The listing builds one solid part. Answer for the finished solid, in the listing's coordinates (mm). A direction names the side the tool comes from. Give positions to 0.01 mm unless a question says otherwise; leave off trailing zeros. Order: outer loops, then holes, each group sorted by start corner. A loop starts at its lowest first (then second) coordinate and runs counter-clockwise, first axis right, second up. Notation, with made-up numbers: (56.5, 22.25) - (92.5, 22.25) arc R23 cw to (92.5, 36.25) - close; hole circle Ø4 at (75, 57.5). An arc over 180 degrees is marked (long way). Answer as a JSON object with one key per item and string values. Group by question number.
Q1. Given pin 1 (6 mm diameter, centred on x = 10, y = 13, fed in from +Z); pin 2 (10 mm diameter, centred on x = 5.5, z = 16, fed in from +Y); pin 3 (8 mm diameter, centred on x = 14.5, z = 6.5, fed in from +Y), each flat-ended and moving along its own axis, determine where each tip first touches the part or whether it passes through.
Q2. Consider line 1 (Z direction, x = 31.5, y = 15); line 2 (Z direction, x = 16, y = 14); line 3 (X direction, y = 23.5, z = 33.5). Determine where each line is inside the solid, lowest interval first.
Q3. For faces 1 (the face through (0, 25, 25)), 2 (the face through (15, 20, 0)), determine the directions among +Z, -Z, +X, -X, +Y, -Y from which every point of the face is accessible in a straight line to the end or side of a thin tool.
Q4. A cutting plane is placed at B-B, the plane y = 38.5. Give the vertices of the cut face in (x, z), and give its area (3 significant figures).
Q5. A cutting plane is placed at A-A, the plane x = 21.5. Give the vertices of the cut face in (y, z).
Q6. The mould has two halves that part along Y. Classify faces 3 (the face through (22.05, 10.82, 14.62)), 4 (the face through (19, 10, 30.365)), 5 (the face through (18.658, 32.88, 11.596)): released by +Y, released by -Y, zero draft, split by the parting line, or undercut.
Q7. A cutting plane is placed at C-C, the plane x = 12.5. Give the vertices of the cut face in (y, z), and give its area (3 significant figures).
Q8. A cutting plane is placed at D-D, the plane x = -1. Give the vertices of the cut face in (y, z).
from build123d import *

# Parameters (mm, degrees)
F0_W     = 40.64
F0_H     = 30.364547
F1_DEPTH = 37.846
F3_DEPTH = 37.847
F4_W     = 49.645454
F4_H     = 41.217271
F5_DEPTH = 9.398
F7_DEPTH = 47.245
F8_R     = 6.184121
F9_DEPTH = 33.775958


with BuildPart() as f1:
    # F0 (on Right) → F1 (new body)
    with BuildSketch(Plane.YZ):
        with Locations((20.32, 15.182273)):
            Rectangle(F0_W, F0_H)
    extrude(amount=F1_DEPTH)

    # F2 (on face) → F3 (cut, through all)
    with BuildSketch(Plane(origin=(0, 0, 0), x_dir=(0, -1, 0), z_dir=(-1, 0, 0))):
        Polygon((-40.64, 0), (-20.32, 30.364547), (-40.64, 30.364547), align=None)
    extrude(amount=-F3_DEPTH, mode=Mode.SUBTRACT)

    # F4 (on face) → F5 (join)
    with BuildSketch(Plane(origin=(0, 0, 0), x_dir=(0, -1, 0), z_dir=(-1, 0, 0))):
        with Locations((-24.822727, 20.608635)):
            Rectangle(F4_W, F4_H)
    extrude(amount=F5_DEPTH)

    # F6 (on face) → F7 (cut, through all)
    with BuildSketch(Plane(origin=(-9.398, 0, 0), x_dir=(0, -1, 0), z_dir=(-1, 0, 0))):
        Polygon((-49.645454, 0), (-24.822727, 41.217271), (-49.645454, 41.217271), align=None)
    extrude(amount=-F7_DEPTH, mode=Mode.SUBTRACT)

    # F8 (on face) → F9 (cut, through all)
    with BuildSketch(Plane(origin=(0, 28.069582, 18.784206), x_dir=(-1, 0, 0), z_dir=(0, 0.831077, 0.556158))):
        with Locations((-21.243637, 0)):
            Circle(F8_R)
    extrude(amount=-F9_DEPTH, mode=Mode.SUBTRACT)


solid = f1.part
Reply:
{
 "1": {"pin 1": "stops at z = 30.36", "pin 2": "stops at y = 33.28", "pin 3": "stops at y = 38.97"},
 "2": {"line 1": "z = 0 to 30.36", "line 2": "z = 0 to 5.42, 13.31 to 30.36", "line 3": "x = -9.4 to 0"},
 "3": {"face 1": "+Z, +X, +Y", "face 2": "-Z, +X, -X, +Y, -Y"},
 "4": {"outline": "(-9.4, 0) - (37.85, 0) - (37.85, 3.2) - (0, 3.2) - (0, 18.51) - (-9.4, 18.51) - close", "area": "295 mm^2"},
 "5": {"outline": "(0, 7.43) - (24.63, 23.92) - (20.32, 30.36) - (0, 30.36) - close; (11.11, 0) - (40.64, 0) - (31.51, 13.65) - close"},
 "6": {"face 3": "undercut", "face 4": "zero draft", "face 5": "released by +Y"},
 "7": {"outline": "(0, 0) - (40.64, 0) - (20.32, 30.36) - (0, 30.36) - close", "area": "926 mm^2"},
 "8": {"outline": "(0, 0) - (49.65, 0) - (24.82, 41.22) - (0, 41.22) - close"}
}
